from build123d import *

# Parameters (mm, degrees)
SKETCH1_R               = 152.4
BOSS_EXTRUDE1_DEPTH     = 76.2
FILLET1_R               = 20
SKETCH2_R               = 15
SKETCH2_R_2             = 7.5
BOSS_EXTRUDE2_DEPTH     = 45
SKETCH4_R               = 3.1
CUT_EXTRUDE1_DEPTH      = 153.4
CUT_EXTRUDE1_DEPTH_BACK = 153.4


with BuildPart() as part:
    # Sketch1 → Boss-Extrude1 (new body)
    with BuildSketch(Plane.XY):
        Circle(SKETCH1_R)
    extrude(amount=BOSS_EXTRUDE1_DEPTH)

    # Fillet1
    fillet1_edges = [part.edges().sort_by_distance(p)[0] for p in [
        (-152.4, 0, 0),
        (-152.4, 0, 76.2),
    ]]
    fillet(fillet1_edges, radius=FILLET1_R)

    # Sketch2 → Boss-Extrude2 (add)
    with BuildSketch(Plane(origin=(0, 0, 0), x_dir=(-1, 0, 0), z_dir=(0, 0, -1))):
        Circle(SKETCH2_R)
        Circle(SKETCH2_R_2, mode=Mode.SUBTRACT)
    extrude(amount=BOSS_EXTRUDE2_DEPTH)

    # Sketch4 → Cut-Extrude1 (cut, two sides)
    with BuildSketch(Plane(origin=(0, 0, 0), x_dir=(0, 0, -1), z_dir=(1, 0, 0))) as cut_extrude1_sk:
        with Locations((30, 0)):
            Circle(SKETCH4_R)
    extrude(amount=CUT_EXTRUDE1_DEPTH, mode=Mode.SUBTRACT)
    extrude(cut_extrude1_sk.sketch, amount=-CUT_EXTRUDE1_DEPTH_BACK, mode=Mode.SUBTRACT)


solid = part.part
Read the model definition and answer for the solid it produces. Units are mm, in the model's axes. A direction names the side the tool comes from. Round coordinates to 2 decimals unless told otherwise and drop trailing zeros. Order: outer loops, then holes, each group sorted by start corner. A loop starts at its lowest first (then second) coordinate and runs counter-clockwise, first axis right, second up.
1) The mould has two halves that part along Y. Classify faces 1 (the face through (-6.93, -2.87, -22.18)), 2 (the face through (-13.856, -5.745, -22.185)), 3 (the face through (28, 2, 0)): released by +Y, released by -Y, zero draft, split by the parting line, or undercut.
2) The part is cut by section D-D on z = 13. Write down the section's boundary in (x, y) (3 decimals), plus the area to 3 significant figures.
3) Straight lines are drawn through the part: L1, parallel to Z at x = -12, y = 0; L2, parallel to X at y = 0, z = -24. For each, find the intervals that lie inside material, in ascending order.
4) For faces 4 (the face through (0, 0, 0)), 5 (the face through (4, 7, -45)), determine the directions among +Z, -Z, +X, -X, +Y, -Y from which every point of the face is accessible in a straight line to the end or side of a thin tool.
5) The part is cut by section C-C on z = 39.5. Write down the section's boundary in (x, y), plus the area to 3 significant figures.
6) The part is cut by section B-B on x = 0. Write down the section's boundary in (y, z), plus the area to 3 significant figures.
7) Flat-ended cylindrical pins translate along their axes: pin 1 (5 mm diameter, centred on y = 0, z = -30, fed in from -X); pin 2 (6 mm diameter, centred on x = -97, y = 3, fed in from -Z); pin 3 (6 mm diameter, centred on y = -69.5, z = 4, fed in from +X); pin 4 (10 mm diameter, centred on y = 87.5, z = 46.5, fed in from +X). Find the tip coordinate at first contact, or state that the pin passes through.
8) The part is cut by section A-A on z = -12.5. Write down the section's boundary in (x, y).
Resolved:
1. face 1: undercut
1. face 2: split by the parting line
1. face 3: zero draft
2. outline: circle Ø302.27 at (0, 0)
2. area: 71,800 mm2
3. L1: z = -45 to -33.1, -26.9 to 76.2
3. L2: x = -15 to -7.5, 7.5 to 15
4. face 4: -Z
4. face 5: -Z, +X, -X, +Y, -Y
5. outline: circle Ø304.8 at (0, 0)
5. area: 73,000 mm2
6. outline: (-152.4, 20) arc R20 ccw to (-132.4, 0) - (-15, 0) - (-15, -45) - (-7.5, -45) - (-7.5, 0) - (7.5, 0) - (7.5, -45) - (15, -45) - (15, 0) - (132.4, 0) arc R20 ccw to (152.4, 20) - (152.4, 56.2) arc R20 ccw to (132.4, 76.2) - (-132.4, 76.2) arc R20 ccw to (-152.4, 56.2) - close
6. area: 23,600 mm2
7. pin 1: passes through
7. pin 2: stops at z = 0
7. pin 3: stops at x = 130.61
7. pin 4: stops at x = 128.14
8. outline: circle Ø30 at (0, 0); hole circle Ø15 at (0, 0)
